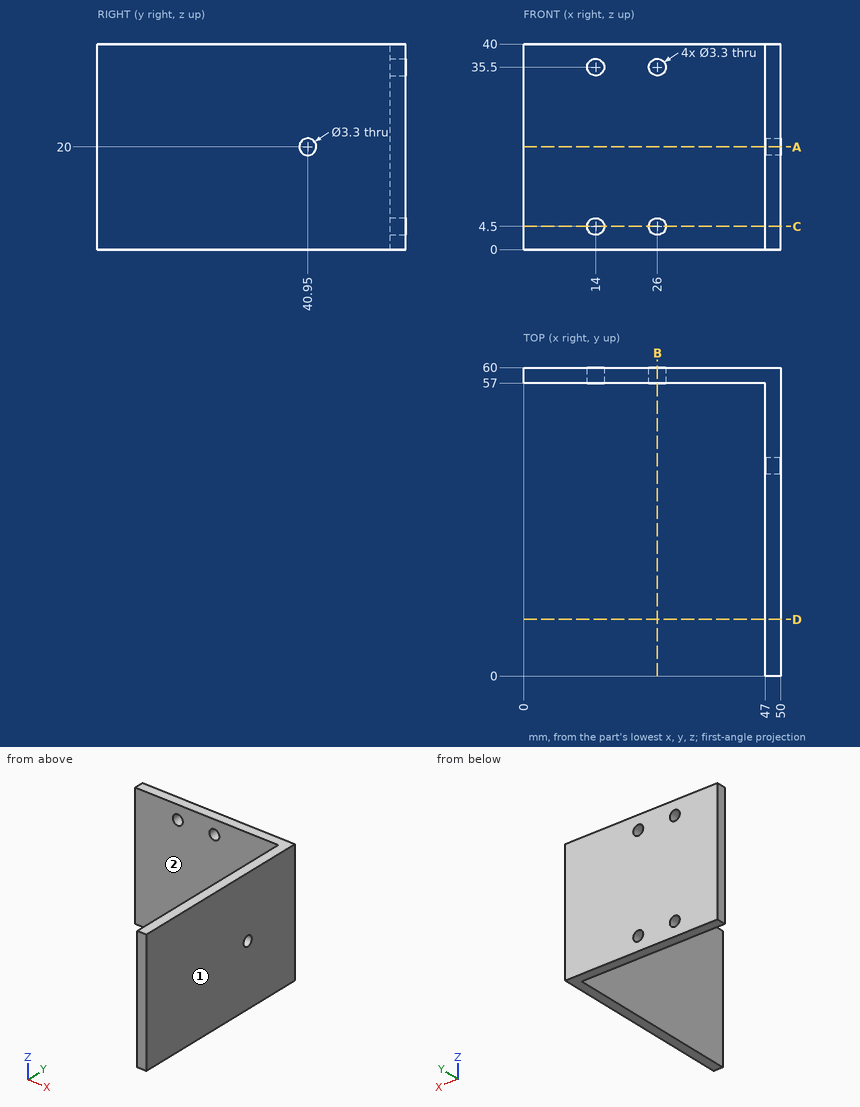
Can you work these out from the drawing? Everything is in mm from the part's minimum corner. A direction names the side the tool comes from. Round coordinates to 2 decimals unless told otherwise and drop trailing zeros. Write each loop counter-clockwise with the first axis right and the second up, starting at its lowest first coordinate (ties: lowest second). Pieces come first, ordered by that corner, then holes. Notation, with made-up numbers: M -14.75,56 L 34.25,56 A19 cw 34.25,82 Z; hole C 7.5,36.5 d4. An arc over 180 degrees is marked long. Use a Markdown table: item, result.
Item 1: I want a section at A-A (z = 20). List the corners of the cut face in (x, y) for me.
Found:
| item | result |
|---|---|
| outline | M 0,57 L 47,57 L 47,42.6 L 50,42.6 L 50,60 L 0,60 Z; M 47,0 L 50,0 L 50,39.3 L 47,39.3 Z |
Item 2: If I drill on line 1 along X through (y, z) = (58.3, 4.5); line 2 along Y through (x, z) = (34, 23.5); line 3 along X through (y, z) = (41, 2.5), over which ranges is the centre line in solid material (lowest first)? Write a range as [from, to].
Found:
| item | result |
|---|---|
| line 1 | x = [0, 12.35], [15.65, 24.35], [27.65, 50] |
| line 2 | y = [57, 60] |
| line 3 | x = [47, 50] |
Item 3: For pin 1 Ø5 at (y, z) = (35, 28) entering from -X; pin 2 Ø12 at (x, z) = (13.5, 24.5) entering from -Y, each with a flat end and sliding along its axis, tell me the tip position at first contact or that it passes through.
Found:
| item | result |
|---|---|
| pin 1 | stops at x = 47 |
| pin 2 | stops at y = 57 |
Item 4: I want a section at D-D (y = 11). List the corners of the cut face in (x, z) for me, and give its area (3 significant figures).
Found:
| item | result |
|---|---|
| outline | M 47,0 L 50,0 L 50,40 L 47,40 Z |
| area | 120 mm2 |
Item 5: I want a section at B-B (x = 26). List the corners of the cut face in (y, z) for me, and give its area (3 significant figures).
Found:
| item | result |
|---|---|
| outline | M 57,0 L 60,0 L 60,2.85 L 57,2.85 Z; M 57,6.15 L 60,6.15 L 60,33.85 L 57,33.85 Z; M 57,37.15 L 60,37.15 L 60,40 L 57,40 Z |
| area | 100 mm2 |
Item 6: I want a section at C-C (z = 4.5). List the corners of the cut face in (x, y) for me.
Found:
| item | result |
|---|---|
| outline | M 0,57 L 12.35,57 L 12.35,60 L 0,60 Z; M 15.65,57 L 24.35,57 L 24.35,60 L 15.65,60 Z; M 27.65,57 L 47,57 L 47,0 L 50,0 L 50,60 L 27.65,60 Z |
Item 7: Which directions (+Z, -Z, +X, -X, +Y, -Y) give clear straight access to the entire face, cutting with the end or side of a thin tool? Please do the marked faces 1 and 2.
Found:
| item | result |
|---|---|
| face 1 | +Z, -Z, +X, +Y, -Y |
| face 2 | +Z, -Z, -X, -Y |
